Input: part model. Units: mm. Frame: model coordinates. Face numbers are marked on the shaded views. A direction names the side the tool comes from. Give positions to 0.01 mm unless a question says otherwise; leave off trailing zeros. Loops run counter-clockwise (first coordinate to the right, second up) from the corner with the lowest first, then second, coordinate; pieces in that order, holes last. Notation, with made-up numbers: (35, 41.5) -> (41, 41.5) arc R15 ccw to (41, 52.5) -> close; hole circle Ø7 at (-40, -29). An arc over 180 degrees is marked (long way). Answer as a JSON object with one key per item and string values.
```python
from build123d import *

# Parameters (mm, degrees)
F1_DEPTH = 52.324
F2_T     = -0.762
F4_D     = 3.2639
F4_DEPTH = 0.762
F4_TIP   = 0.9805744872
F6_D     = 3.2639
F8_D     = 3.2639
F8_DEPTH = 0.762
F8_TIP   = 0.9805744872


with BuildPart() as f1:
    # F0 (on Top) → F1 (new body)
    with BuildSketch(Plane.XY):
        Polygon((0, 181.61), (-181.61, 181.61), (-181.61, -181.61), (0, -181.61), (0, 0), align=None)
        Polygon((181.61, 181.61), (0, 181.61), (0, 0), (0, -181.61), (181.61, -181.61), align=None)
    extrude(amount=F1_DEPTH)

    # F2
    f2_openings = [f1.faces().sort_by_distance(p)[0] for p in [
        (0, 0, 0),
    ]]
    offset(amount=F2_T, openings=f2_openings)

    # F4
    with Locations(Plane.XZ.offset(181.61)):
        with Locations((-139.7, 7.112), (0, 7.112), (139.7, 7.112)):
            Hole(F4_D / 2, depth=F4_DEPTH)
            with Locations((0, 0, -(F4_DEPTH + F4_TIP / 2))):  # 118° drill point
                Cone(0, F4_D / 2, F4_TIP, mode=Mode.SUBTRACT)

    # F6 (through all)
    with Locations(Plane(origin=(-181.61, 0, 0), x_dir=(0, -1, 0), z_dir=(-1, 0, 0))):
        with Locations((-139.7, 7.112), (0, 7.112), (139.7, 7.112)):
            Hole(F6_D / 2)

    # F8
    with Locations(Plane(origin=(0, 181.61, 0), x_dir=(-1, 0, 0), z_dir=(0, 1, 0))):
        with Locations((-127, 19.05), (-63.5, 19.05), (0, 19.05), (63.5, 19.05), (127, 19.05)):
            Hole(F8_D / 2, depth=F8_DEPTH)
            with Locations((0, 0, -(F8_DEPTH + F8_TIP / 2))):  # 118° drill point
                Cone(0, F8_D / 2, F8_TIP, mode=Mode.SUBTRACT)


solid = f1.part
```
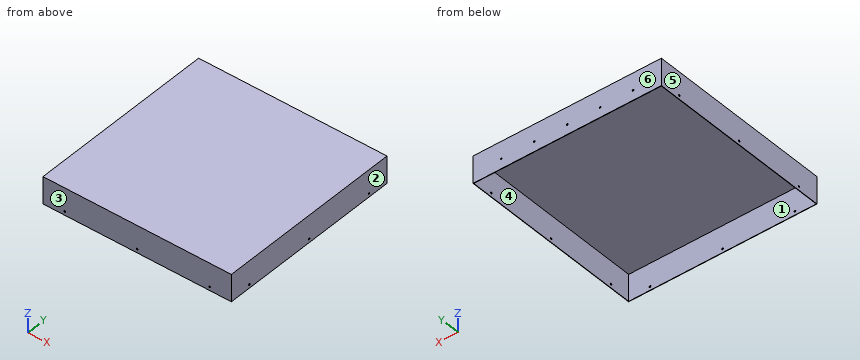
Q1. Draft query along Y for the marked faces 3, 4, 5 and 6. Return one class per face: +Y half, -Y half, draft (parallel to the pull), parting line (faces both ways), or undercut.
Evaluation:
{"face 3": "-Y half", "face 4": "undercut", "face 5": "draft", "face 6": "+Y half"}
Q2. Ray query, line 1 along X through (y, z) = (-90, 34); line 2 along Z through (x, y) = (181.2, 139.7). Return the intervals inside material, ascending.
Evaluation:
{"line 1": "x = -181.61 to -180.85, 180.85 to 181.61", "line 2": "z = 0 to 5.48, 8.74 to 52.32"}
Q3. Pin query (flat end, axial travel): pin 1 (2 mm diameter, centred on x = 127, y = 7.5, fed in from -Z). Return the tip coordinate at first contact, or that it passes through.
Evaluation:
{"pin 1": "stops at z = 51.56"}
Q4. Section C-C, the plane z = 46.5. Return the cut outline in (x, y).
Evaluation:
{"outline": "(-181.61, -181.61) -> (181.61, -181.61) -> (181.61, 181.61) -> (-181.61, 181.61) -> close; hole (-180.85, -180.85) -> (180.85, -180.85) -> (180.85, 180.85) -> (-180.85, 180.85) -> close"}
Q5. Section A-A, the plane x = 35. Return the cut outline in (y, z).
Evaluation:
{"outline": "(-181.61, 0) -> (-180.85, 0) -> (-180.85, 51.56) -> (180.85, 51.56) -> (180.85, 0) -> (181.61, 0) -> (181.61, 52.32) -> (-181.61, 52.32) -> close"}
Q6. Access query for the marked faces 1 and 2. Directions: +Z, -Z, +X, -X, +Y, -Y. A direction counts if a zero-diameter tool reaches every point of the face in a straight line with its end or side. Return the directions, or none.
Evaluation:
{"face 1": "-Z", "face 2": "+Z, -Z, +X, +Y, -Y"}
